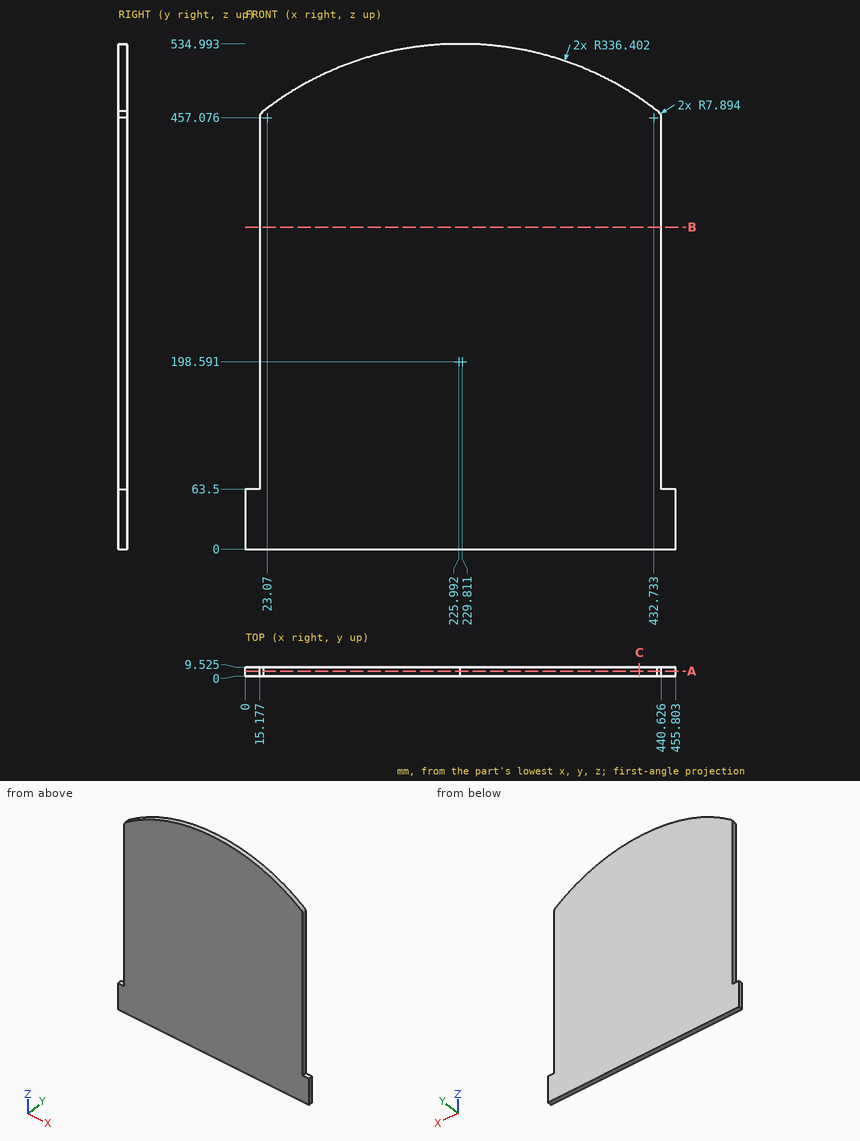
The figure shows three views and two pictorial views of one solid part (mm, origin at its lowest corner). Answer the questions. Coordinates: 2 decimals unless noted, no trailing zeros. Loops run counter-clockwise (first coordinate to the right, second up) from the corner with the lowest first, then second, coordinate; pieces in that order, holes last. Notation, with made-up numbers: (-9, 83) - (31, 83) arc R34 ccw to (31, 116) - close; hole circle Ø11 at (82, 23). An arc over 180 degrees is marked (long way). Use a Markdown table: item, result. Add a question column.
1) Given pin 1 (3 mm diameter, centred on x = 10, y = 7, fed in from +Z); pin 2 (3 mm diameter, centred on y = 6.5, z = 374.5, fed in from -X); pin 3 (3 mm diameter, centred on y = 3.5, z = 318, fed in from +X), each flat-ended and moving along its own axis, determine where each tip first touches the part or whether it passes through.
2) The part is cut by section A-A, the plane y = 5.25. Give the vertices of the cut face in (x, z) (1 decimal), and give its area (3 significant figures).
3) The part is cut by section C-C, the plane x = 417.5. Give the vertices of the cut face in (y, z) (1 decimal), and give its area (3 significant figures).
4) Find the intervals of material crossed by line 1 (X direction, y = 1, z = 330); line 2 (Z direction, x = 225, y = 4); line 3 (Z direction, x = 143, y = 4.25) (1 decimal), in increasing order.
5) The part is cut by section B-B, the plane z = 341. Give the vertices of the cut face in (x, y) (1 decimal), and give its area (3 significant figures).
Here are the results:
| question | item | result |
|---|---|---|
| 1 | pin 1 | stops at z = 63.5 |
| 1 | pin 2 | stops at x = 15.18 |
| 1 | pin 3 | stops at x = 440.63 |
| 2 | outline | (0, 0) - (455.8, 0) - (455.8, 63.5) - (440.6, 63.5) - (440.6, 457.2) arc R7.9 ccw to (436.5, 464) arc R336.4 ccw to (227.9, 535) arc R336.4 ccw to (19.3, 464) arc R7.9 ccw to (15.2, 457.2) - (15.2, 63.5) - (0, 63.5) - close |
| 2 | area | 220,000 mm^2 |
| 3 | outline | (0, 0) - (9.5, 0) - (9.5, 477.8) - (0, 477.8) - close |
| 3 | area | 4,550 mm^2 |
| 4 | line 1 | x = 15.18 to 440.63 |
| 4 | line 2 | z = 0 to 534.99 |
| 4 | line 3 | z = 0 to 524.6 |
| 5 | outline | (15.2, 0) - (440.6, 0) - (440.6, 9.5) - (15.2, 9.5) - close |
| 5 | area | 4,050 mm^2 |
